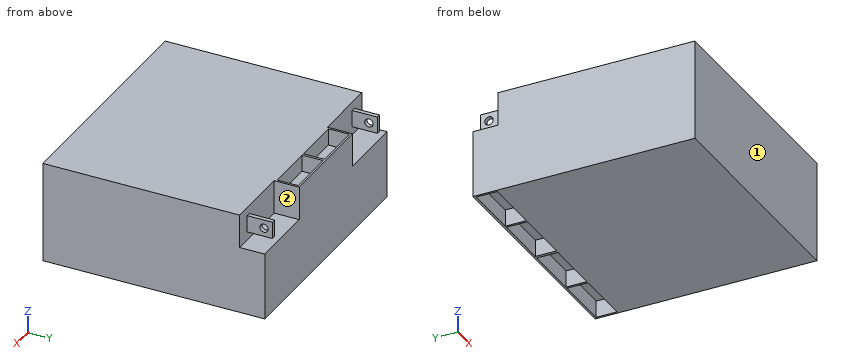
Autodesk Inventor part; units mm, degrees
ref_plane "YZ Plane" through (0, 0, 0) normal (1, 0, 0) x (0, 1, 0)
ref_plane "XZ Plane" through (0, 0, 0) normal (0, 1, 0) x (-1, 0, 0)
ref_plane "XY Plane" through (0, 0, 0) normal (0, 0, 1) x (1, 0, 0)
sketch "Sketch1" plane through (0, 0, 0) normal (0, 1, 0) x (-1, 0, 0)
  line L0 (0, 0) -> (-180.34, 0)
  line L1 (-180.34, 0) -> (-180.34, -76.2)
  line L2 (-180.34, -76.2) -> (0, -76.2)
  line L3 (0, -76.2) -> (0, 0)
  dimension "d0" = 180.34
  dimension "d1" = 76.2
extrude "Extrusion1" add sketch "Sketch1" along normal blind 167.64
sketch "Sketch2" plane through (0, 167.64, 0) normal (0, 1, 0) x (1, 0, 0)
  line L0 (0, 0) -> (180.34, 0)
  line L1 (180.34, 0) -> (180.34, 76.2)
  line L2 (180.34, 76.2) -> (0, 76.2)
  line L3 (0, 76.2) -> (0, 0)
  line L4 (0, 0) -> (50.8, 0)
  line L5 (50.8, 0) -> (50.8, 25.4)
  line L6 (50.8, 25.4) -> (0, 25.4)
  line L7 (0, 25.4) -> (0, 0)
  line L8 (180.34, 0) -> (129.54, 0)
  line L9 (129.54, 0) -> (129.54, 25.4)
  line L10 (129.54, 25.4) -> (180.34, 25.4)
  line L11 (180.34, 25.4) -> (180.34, 0)
  dimension "d4" = 50.8
  dimension "d5" = 25.4
  dimension "d6" = 50.8
  dimension "d7" = 25.4
extrude "Extrusion2" cut sketch "Sketch2" against normal blind 19.05 contours L3 L6 L5 L0 | L9 L10 L1 L0
sketch "Sketch3" plane through (0, 0, 0) normal (0, 0, 1) x (1, 0, 0)
  line L0 (50.8, 167.64) -> (50.8, 148.59) construction
  line L1 (50.8, 148.59) -> (0, 148.59)
  line L2 (0, 0) -> (0, 148.59)
  line L3 (0, 0) -> (180.34, 0)
  line L4 (180.34, 0) -> (180.34, 148.59)
  line L5 (180.34, 148.59) -> (129.54, 148.59)
  line L6 (129.54, 148.59) -> (129.54, 167.64) construction
  line L7 (50.8, 167.64) -> (129.54, 167.64) construction
  line L8 (50.8, 167.64) -> (129.54, 167.64)
  line L9 (129.54, 167.64) -> (129.54, 148.59)
  line L10 (129.54, 148.59) -> (50.8, 148.59) construction
  line L11 (50.8, 148.59) -> (50.8, 167.64)
  line L12 (52.3875, 150.1775) -> (127.9525, 150.1775) construction
  line L13 (127.9525, 150.1775) -> (127.9525, 166.0525) construction
  line L14 (127.9525, 166.0525) -> (52.3875, 166.0525) construction
  line L15 (52.3875, 166.0525) -> (52.3875, 150.1775) construction
  line L16 (52.3875, 166.0525) -> (89.2175, 166.0525)
  line L17 (89.2175, 166.0525) -> (89.2175, 150.1775)
  line L18 (89.2175, 150.1775) -> (52.3875, 150.1775)
  line L19 (52.3875, 150.1775) -> (52.3875, 166.0525)
  line L20 (127.9525, 150.1775) -> (91.1225, 150.1775)
  line L21 (91.1225, 150.1775) -> (91.1225, 166.0525)
  line L22 (91.1225, 166.0525) -> (127.9525, 166.0525)
  line L23 (127.9525, 166.0525) -> (127.9525, 150.1775)
  dimension "d10" = 1.5875
  dimension "d11" = 36.83
  dimension "d12" = 36.83
extrude "Extrusion3" cut sketch "Sketch3" against normal blind 12.7 contours L16 L17 L18 L19 | L20 L21 L22 L23
sketch "Sketch4" plane through (180.34, 0, -76.2) normal (0, 0, -1) x (-1, 0, 0)
  line L0 (0, 0) -> (180.34, 0) construction
  line L1 (180.34, 0) -> (180.34, 167.64) construction
  line L2 (0, 167.64) -> (180.34, 167.64) construction
  line L3 (0, 0) -> (0, 167.64) construction
  line L4 (0, 167.64) -> (180.34, 167.64) construction
  line L5 (180.34, 167.64) -> (180.34, 148.59) construction
  line L6 (180.34, 148.59) -> (0, 148.59) construction
  line L7 (0, 148.59) -> (0, 167.64) construction
  line L8 (1.5875, 150.1775) -> (178.7525, 150.1775) construction
  line L9 (178.7525, 150.1775) -> (178.7525, 166.0525) construction
  line L10 (178.7525, 166.0525) -> (1.5875, 166.0525) construction
  line L11 (1.5875, 166.0525) -> (1.5875, 150.1775) construction
  line L12 (1.5875, 166.0525) -> (44.5135, 166.0525)
  line L13 (44.5135, 166.0525) -> (44.5135, 150.1775)
  line L14 (44.5135, 150.1775) -> (1.5875, 150.1775)
  line L15 (1.5875, 150.1775) -> (1.5875, 166.0525)
  line L16 (178.7525, 150.1775) -> (135.8265, 150.1775)
  line L17 (135.8265, 150.1775) -> (135.8265, 166.0525)
  line L18 (135.8265, 166.0525) -> (178.7525, 166.0525)
  line L19 (178.7525, 166.0525) -> (178.7525, 150.1775)
  line L20 (46.101, 150.1775) -> (89.027, 150.1775)
  line L21 (89.027, 150.1775) -> (89.027, 166.0525)
  line L22 (89.027, 166.0525) -> (46.101, 166.0525)
  line L23 (46.101, 166.0525) -> (46.101, 150.1775)
  line L24 (134.239, 150.1775) -> (91.313, 150.1775)
  line L25 (91.313, 150.1775) -> (91.313, 166.0525)
  line L26 (91.313, 166.0525) -> (134.239, 166.0525)
  line L27 (134.239, 166.0525) -> (134.239, 150.1775)
  dimension "d15" = 1.5875
  dimension "d16" = 42.926
  dimension "d17" = 42.926
  dimension "d18" = 42.926
  dimension "d19" = 42.926
  dimension "d20" = 1.5875
  dimension "d21" = 1.5875
extrude "Extrusion4" cut sketch "Sketch4" against normal blind 12.7
sketch "Sketch5" plane through (0, 148.59, 0) normal (0, 1, 0) x (1, 0, 0)
  line L0 (50.8, 0) -> (0, 0)
  line L1 (50.8, 25.4) -> (50.8, 0)
  line L2 (0, 25.4) -> (50.8, 25.4)
  line L3 (0, 0) -> (0, 25.4)
  line L4 (180.34, 25.4) -> (180.34, 0)
  line L5 (129.54, 25.4) -> (180.34, 25.4)
  line L6 (129.54, 0) -> (129.54, 25.4)
  line L7 (180.34, 0) -> (129.54, 0)
  line L8 (0, 0) -> (12.7, 0) construction
  line L9 (12.7, 0) -> (12.7, 12.7) construction
  line L10 (12.7, 12.7) -> (0, 12.7) construction
  line L11 (0, 12.7) -> (0, 0) construction
  line L12 (180.34, 0) -> (167.64, 0) construction
  line L13 (167.64, 0) -> (167.64, 12.7) construction
  line L14 (167.64, 12.7) -> (180.34, 12.7) construction
  line L15 (180.34, 12.7) -> (180.34, 0) construction
  line L16 (11.1125, 19.05) -> (14.2875, 19.05)
  line L17 (14.2875, 19.05) -> (14.2875, 6.35)
  line L18 (14.2875, 6.35) -> (11.1125, 6.35)
  line L19 (11.1125, 6.35) -> (11.1125, 19.05)
  line L20 (11.1125, 19.05) -> (14.2875, 6.35) construction
  line L21 (14.2875, 19.05) -> (11.1125, 6.35) construction
  line L22 (169.2275, 6.35) -> (166.0525, 6.35)
  line L23 (166.0525, 6.35) -> (166.0525, 19.05)
  line L24 (166.0525, 19.05) -> (169.2275, 19.05)
  line L25 (169.2275, 19.05) -> (169.2275, 6.35)
  line L26 (169.2275, 6.35) -> (166.0525, 19.05) construction
  line L27 (166.0525, 6.35) -> (169.2275, 19.05) construction
  dimension "d24" = 12.7
  dimension "d25" = 12.7
  dimension "d26" = 12.7
  dimension "d27" = 12.7
  dimension "d28" = 3.175
  dimension "d29" = 12.7
  dimension "d30" = 3.175
  dimension "d31" = 12.7
extrude "Extrusion5" add sketch "Sketch5" along normal blind 19.05 contours L16 L17 L18 L19 | L22 L23 L24 L25
sketch "Sketch6" plane through (169.2275, 148.59, -6.35) normal (1, 0, 0) x (0, 0, -1)
  line L0 (12.7, 0) -> (0, 0) construction
  line L1 (12.7, 0) -> (12.7, 19.05) construction
  line L2 (0, 19.05) -> (12.7, 19.05) construction
  line L3 (0, 0) -> (0, 19.05) construction
  line L4 (0, 19.05) -> (6.35, 19.05) construction
  line L5 (6.35, 19.05) -> (6.35, 12.7) construction
  line L6 (6.35, 12.7) -> (0, 12.7) construction
  line L7 (0, 12.7) -> (0, 19.05) construction
  circle A0 centre (6.35, 12.7) radius 3.175
  point P0 (-6.35, -148.59)
  dimension "d34" = 6.35
  dimension "d35" = 6.35
  dimension "d36" = 6.35
extrude "Extrusion6" cut sketch "Sketch6" against normal blind 25.4
sketch "Sketch7" plane through (11.1125, 148.59, -19.05) normal (-1, 0, 0) x (0, 0, 1)
  line L0 (12.7, 0) -> (0, 0) construction
  line L1 (12.7, 0) -> (12.7, 19.05) construction
  line L2 (0, 19.05) -> (12.7, 19.05) construction
  line L3 (0, 0) -> (0, 19.05) construction
  line L4 (12.7, 19.05) -> (6.35, 19.05) construction
  line L5 (6.35, 19.05) -> (6.35, 12.7) construction
  line L6 (6.35, 12.7) -> (12.7, 12.7) construction
  line L7 (12.7, 12.7) -> (12.7, 19.05) construction
  circle A0 centre (6.35, 12.7) radius 3.175
  point P0 (19.05, -148.59)
  dimension "d39" = 6.35
  dimension "d40" = 6.35
  dimension "d41" = 6.35
extrude "Extrusion7" cut sketch "Sketch7" against normal blind 25.4
properties part number "battery"
CAD build for the part. Positions are in the model's coordinates, mm. Face numbers are marked on the shaded views. A direction names the side the tool comes from. Round coordinates to 2 decimals unless told otherwise and drop trailing zeros. Write each loop counter-clockwise with the first axis right and the second up, starting at its lowest first coordinate (ties: lowest second). Pieces come first, ordered by that corner, then holes. Notation, with made-up numbers: (8, 16) -> (29, 16) arc R11 ccw to (29, 33) -> close; hole circle Ø3 at (28.25, -19). An arc over 180 degrees is marked (long way). Answer in a Markdown table with one row per item. Add a question column.
Item 1: Saw through at A-A, the plane y = 161.29. Count the separate pieces of the cut face and the enclosed holes in it, then the cut area to 3 significant figures.
Item 2: Saw through at B-B, the plane x = 107. Write the cut outline in (y, z), then the cut area to 3 significant figures.
Item 3: Drill centre lines: line 1 (Z direction, x = 12, y = 161); line 2 (Y direction, x = 167.25, z = -12.7) (3 decimals); line 3 (Y direction, x = 9, z = -65). Where is each one in solid material? Low to high. Write a range as from..to.
Item 4: Drop flat-ended pins along their axis: pin 1 Ø5.5 at (y, z) = (158.5, -17.5) entering from +X; pin 2 Ø4 at (y, z) = (161.29, -12.7) entering from -X; pin 3 Ø10 at (y, z) = (154.5, -8) entering from -X. Give the stop position or say it passes through.
Item 5: Saw through at C-C, the plane x = 152. Write the cut outline in (y, z), then the cut area to 3 significant figures.
Item 6: Which spindle directions (+Z, -Z, +X, -X, +Y, -Y) get a long thin tool onto all of the face, cutting with end or side? Do the marked faces 1 and 2. Say none if no direction does.
Findings below:
| question | item | result |
|---|---|---|
| 1 | separate pieces | 5 |
| 1 | enclosed holes | 0 |
| 1 | area | 8,090 mm^2 |
| 2 | outline | (0, -76.2) -> (150.18, -76.2) -> (150.18, -63.5) -> (166.05, -63.5) -> (166.05, -76.2) -> (167.64, -76.2) -> (167.64, 0) -> (166.05, 0) -> (166.05, -12.7) -> (150.18, -12.7) -> (150.18, 0) -> (0, 0) -> close |
| 2 | area | 12,400 mm^2 |
| 3 | line 1 | z = -63.5..-25.4, -19.05..-15.86, -9.54..-6.35 |
| 3 | line 2 | y = 0..158.115, 164.465..167.64 |
| 3 | line 3 | y = 0..150.18, 166.05..167.64 |
| 4 | pin 1 | stops at x = 169.23 |
| 4 | pin 2 | stops at x = 50.8 |
| 4 | pin 3 | stops at x = 11.11 |
| 5 | outline | (0, -76.2) -> (150.18, -76.2) -> (150.18, -63.5) -> (166.05, -63.5) -> (166.05, -76.2) -> (167.64, -76.2) -> (167.64, -25.4) -> (148.59, -25.4) -> (148.59, 0) -> (0, 0) -> close |
| 5 | area | 12,100 mm^2 |
| 6 | face 1 | +Z, -Z, +X, -X, -Y |
| 6 | face 2 | +Z, +Y |
